Part print with two shaded views. Sizes in mm from the minimum x, y, z corner. A direction names the side the tool comes from. Round coordinates to 2 decimals unless told otherwise and drop trailing zeros. Write each loop counter-clockwise with the first axis right and the second up, starting at its lowest first coordinate (ties: lowest second). Pieces come first, ordered by that corner, then holes. Notation, with made-up numbers: (7.25, 55) -> (39.25, 55) arc R28 ccw to (39.25, 81) -> close; hole circle Ø6 at (12.5, 23.5). An arc over 180 degrees is marked (long way). Answer in a Markdown table with one row per item.
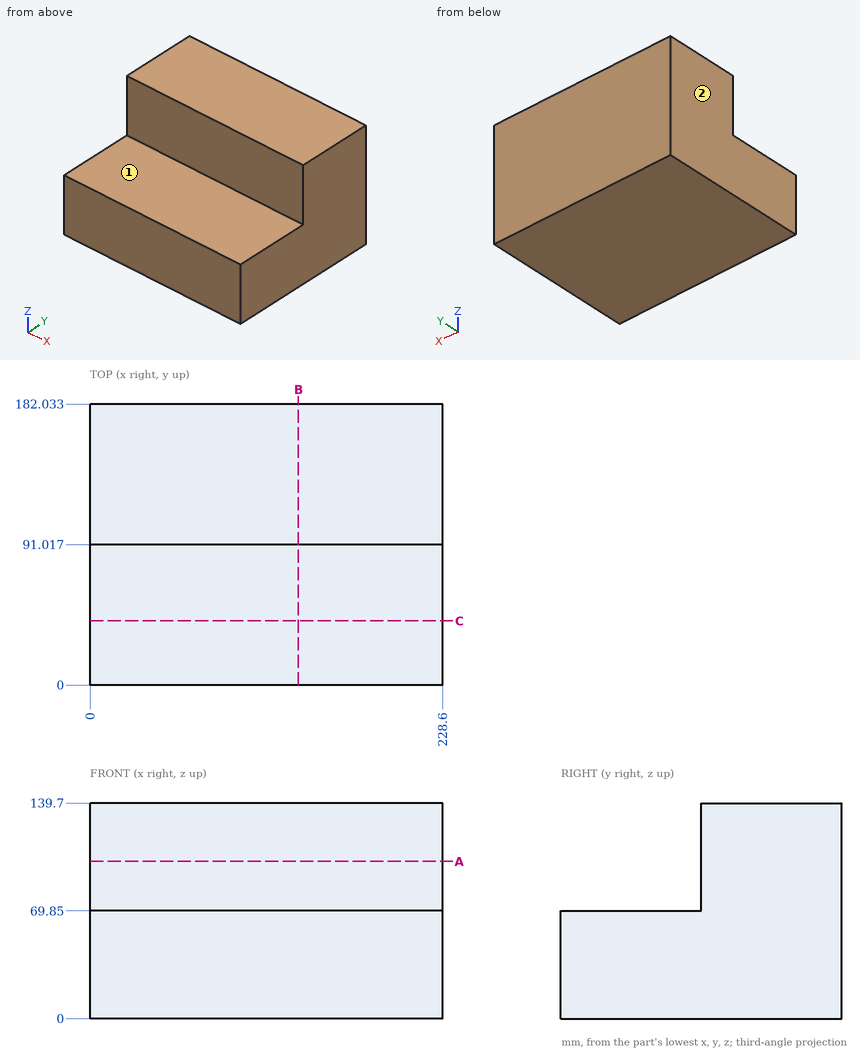
Q1. Drop flat-ended pins along their axis: P1, Ø12, axis at x = 93, y = 50.5, coming from the +Z side; P2, Ø21, axis at x = 65.5, z = 108, coming from the -Y side. Give the stop position or say it passes through.
A:
| item | result |
|---|---|
| P1 | z = 69.85 |
| P2 | y = 91.02 |
Q2. Saw through at A-A on z = 102. Write the cut outline in (x, y), plus the area to 3 significant figures.
A:
| item | result |
|---|---|
| outline | (0, 91.02) -> (228.6, 91.02) -> (228.6, 182.03) -> (0, 182.03) -> close |
| area | 20,800 mm² |
Q3. Wall check: line 1 (Z direction, x = 38, y = 16); line 2 (Y direction, x = 78.5, z = 99). Give the ranges that are in metal, low to high. Write a range as [from, to].
A:
| item | result |
|---|---|
| line 1 | [0, 69.85] |
| line 2 | [91.02, 182.03] |
Q4. Which spindle directions (+Z, -Z, +X, -X, +Y, -Y) get a long thin tool onto all of the face, cutting with end or side? Do the marked faces 1 and 2. Say none if no direction does.
A:
| item | result |
|---|---|
| face 1 | +Z, +X, -X, -Y |
| face 2 | +Z, -Z, -X, +Y, -Y |
Q5. Saw through at C-C on y = 41.5. Write the cut outline in (x, z).
A:
| item | result |
|---|---|
| outline | (0, 0) -> (228.6, 0) -> (228.6, 69.85) -> (0, 69.85) -> close |
Q6. Saw through at B-B on x = 135. Write the cut outline in (y, z).
A:
| item | result |
|---|---|
| outline | (0, 0) -> (182.03, 0) -> (182.03, 139.7) -> (91.02, 139.7) -> (91.02, 69.85) -> (0, 69.85) -> close |
